Geometry: final body of the model. Coordinates: model frame, mm. A direction names the side the tool comes from. Coordinates: 2 decimals unless noted, no trailing zeros. Loops run counter-clockwise (first coordinate to the right, second up) from the corner with the lowest first, then second, coordinate; pieces in that order, holes last. Notation, with made-up numbers: (74.5, -36) - (81.5, -36) arc R16 ccw to (81.5, -21) - close; hole circle Ø7 at (45, 75). An arc over 180 degrees is marked (long way). Write each question's results on one line, items separated by ' | '. Start each with the question number.
from build123d import *

# Parameters (mm, degrees)
SKETCH1_W               = 12
SKETCH1_H               = 12
SKETCH1_R               = 5.5
BOSS_EXTRUDE1_DEPTH     = 6
BOSS_EXTRUDE1_2_DEPTH   = 6
BOSS_EXTRUDE1_3_DEPTH   = 6
BOSS_EXTRUDE1_4_DEPTH   = 6
BOSS_EXTRUDE1_5_DEPTH   = 6
BOSS_EXTRUDE1_6_DEPTH   = 6
BOSS_EXTRUDE2_START     = -6
BOSS_EXTRUDE2_OUTLINE_R = 1.7
BOSS_EXTRUDE2_DEPTH     = 6
CUT_EXTRUDE1_DEPTH      = 1


# Read off the part's stored shape, not the designer's step: Boss-Extrude2
with BuildPart() as part:
    # Sketch1 → Boss-Extrude1 (new body)
    with BuildSketch(Plane(origin=(0, 0, 0), x_dir=(1, 0, 0), z_dir=(0, 1, 0))):
        with Locations((-2.713611414, -10.664883528)):
            Rectangle(SKETCH1_W, SKETCH1_H)
        with Locations(Location((-2.713611414, -10.664883528, 0), (0, 0, 270))):
            Circle(SKETCH1_R, mode=Mode.SUBTRACT)
    extrude(amount=-BOSS_EXTRUDE1_DEPTH)



with BuildPart() as body_2:
    # Sketch1 → Boss-Extrude1 2 (new body)
    with BuildSketch(Plane(origin=(0, 0, 0), x_dir=(1, 0, 0), z_dir=(0, 1, 0))):
        with Locations((12.886388586, -10.664882884)):
            Rectangle(SKETCH1_W, SKETCH1_H)
        with Locations(Location((12.886388586, -10.664882884, 0), (0, 0, 270))):
            Circle(SKETCH1_R, mode=Mode.SUBTRACT)
    extrude(amount=-BOSS_EXTRUDE1_2_DEPTH)


with BuildPart() as body_3:
    # Sketch1 → Boss-Extrude1 3 (new body)
    with BuildSketch(Plane(origin=(0, 0, 0), x_dir=(1, 0, 0), z_dir=(0, 1, 0))):
        with Locations((5.086388588, -23.66488245)):
            Rectangle(SKETCH1_W, SKETCH1_H)
        with Locations(Location((5.086388588, -23.66488245, 0), (0, 0, 270))):
            Circle(SKETCH1_R, mode=Mode.SUBTRACT)
    extrude(amount=-BOSS_EXTRUDE1_3_DEPTH)


with BuildPart() as body_4:
    # Sketch1 → Boss-Extrude1 4 (new body)
    with BuildSketch(Plane(origin=(0, 0, 0), x_dir=(1, 0, 0), z_dir=(0, 1, 0))):
        with Locations((20.686388588, -23.664882884)):
            Rectangle(SKETCH1_W, SKETCH1_H)
        with Locations(Location((20.686388588, -23.664882884, 0), (0, 0, 270))):
            Circle(SKETCH1_R, mode=Mode.SUBTRACT)
    extrude(amount=-BOSS_EXTRUDE1_4_DEPTH)


with BuildPart() as body_5:
    # Sketch1 → Boss-Extrude1 5 (new body)
    with BuildSketch(Plane(origin=(0, 0, 0), x_dir=(1, 0, 0), z_dir=(0, 1, 0))):
        with Locations((28.486388586, -10.664882884)):
            Rectangle(SKETCH1_W, SKETCH1_H)
        with Locations(Location((28.486388586, -10.664882884, 0), (0, 0, 270))):
            Circle(SKETCH1_R, mode=Mode.SUBTRACT)
    extrude(amount=-BOSS_EXTRUDE1_5_DEPTH)


with BuildPart() as body_6:
    # Sketch1 → Boss-Extrude1 6 (new body)
    with BuildSketch(Plane(origin=(0, 0, 0), x_dir=(1, 0, 0), z_dir=(0, 1, 0))):
        with Locations((36.286388588, -23.664883087)):
            Rectangle(SKETCH1_W, SKETCH1_H)
        with Locations(Location((36.286388588, -23.664883087, 0), (0, 0, 270))):
            Circle(SKETCH1_R, mode=Mode.SUBTRACT)
    extrude(amount=-BOSS_EXTRUDE1_6_DEPTH)


with BuildPart() as part_1:
    add(part.part)

    add(body_2.part)  # Boss-Extrude2 merges body 2

    add(body_3.part)  # Boss-Extrude2 merges body 3

    add(body_4.part)  # Boss-Extrude2 merges body 4

    add(body_5.part)  # Boss-Extrude2 merges body 5

    add(body_6.part)  # Boss-Extrude2 merges body 6
    # Boss-Extrude2 outline → Boss-Extrude2 (add)
    with BuildSketch(Plane(origin=(0, 0, 0), x_dir=(1, 0, 0), z_dir=(0, 1, 0)).offset(BOSS_EXTRUDE2_START)):
        Polygon((23.186388588, -30.164882884), (33.786388588, -30.164882884), (33.786388588, -29.664883087), (30.286388588, -29.664883087), (30.286388588, -17.664883087), (42.286388588, -17.664883087), (42.286388588, -29.664883087), (38.786388588, -29.664883087), (38.786388588, -30.164883087), (54.418988347, -30.16488245), (54.418988347, -4.164883528), (30.986388586, -4.164882884), (30.986388586, -4.664882884), (34.486388586, -4.664882884), (34.486388586, -16.664882884), (22.486388586, -16.664882884), (22.486388586, -4.664882884), (25.986388586, -4.664882884), (25.986388586, -4.164882884), (15.386388586, -4.164882884), (15.386388586, -4.664882884), (18.886388586, -4.664882884), (18.886388586, -16.664882884), (6.886388586, -16.664882884), (6.886388586, -4.664882884), (10.386388586, -4.664882884), (10.386388586, -4.164882884), (-0.213611414, -4.164883528), (-0.213611414, -4.664883528), (3.286388586, -4.664883528), (3.286388586, -16.664883528), (-8.713611414, -16.664883528), (-8.713611414, -4.664883528), (-5.213611414, -4.664883528), (-5.213611414, -4.164883528), (-19.213611414, -4.164883528), (-19.213611414, -30.16488245), (2.586388588, -30.16488245), (2.586388588, -29.66488245), (-0.913611412, -29.66488245), (-0.913611412, -17.66488245), (11.086388588, -17.66488245), (11.086388588, -29.66488245), (7.586388588, -29.66488245), (7.586388588, -30.16488245), (18.186388588, -30.164882884), (18.186388588, -29.664882884), (14.686388588, -29.664882884), (14.686388588, -17.664882884), (26.686388588, -17.664882884), (26.686388588, -29.664882884), (23.186388588, -29.664882884), align=None)
        with Locations((-14.213611414, -17.164882989)):
            Circle(BOSS_EXTRUDE2_OUTLINE_R, mode=Mode.SUBTRACT)
        with Locations((49.418988347, -17.164882989)):
            Circle(BOSS_EXTRUDE2_OUTLINE_R, mode=Mode.SUBTRACT)
    extrude(amount=BOSS_EXTRUDE2_DEPTH)

    # Sketch2 → Cut-Extrude1 (cut)
    with BuildSketch(Plane(origin=(0, -6, 0), x_dir=(-1, 0, 0), z_dir=(0, -1, 0))):
        Polygon((6.798219501, -22.292392997), (8.345014372, -22.292392997), (8.345014372, -22.618034023), (7.083155398, -22.618034023), (7.083155398, -23.5949571), (8.345014372, -23.5949571), (8.345014372, -23.920598125), (7.083155398, -23.920598125), (7.083155398, -25.467392997), (6.798219501, -25.467392997), align=None)
        with BuildLine():
            Line((10.624501552, -22.292392997), (10.624501552, -22.618034023))
            Line((10.624501552, -22.618034023), (9.545179637, -22.618034023))
            Line((9.545179637, -22.618034023), (9.373454877, -23.453125169))
            add(Edge.make_bspline(
                [(9.373454877, -23.453125169), (9.407069849, -23.443844851), (9.47219354, -23.425865702), (9.568314271, -23.405903325), (9.65956577, -23.393869672), (9.718779856, -23.392226555), (9.747433243, -23.391431459)],
                knots=[0, 0, 0, 0, 1.100273476, 2.13160584, 3.095893838, 4, 4, 4, 4], degree=3))
            add(Edge.make_bspline(
                [(9.747433243, -23.391431459), (9.782887778, -23.392198843), (9.852600253, -23.393707713), (9.95459844, -23.408196462), (10.051964708, -23.431001956), (10.144495429, -23.462861287), (10.232361786, -23.50360083), (10.314755359, -23.55449149), (10.392912895, -23.613939584), (10.465432248, -23.682288273), (10.531222156, -23.757510025), (10.589067018, -23.838388951), (10.638200225, -23.924139045), (10.677716053, -24.015579597), (10.709270413, -24.111699686), (10.73027258, -24.213510672), (10.744257737, -24.320052895), (10.745820188, -24.392900612), (10.746616936, -24.430048246)],
                knots=[0, 0, 0, 0, 1.052922333, 2.070308379, 3.05430497, 4.020497103, 4.973039431, 5.925935799, 6.892292201, 7.88610001, 8.88166317, 9.857072816, 10.836096531, 11.812156883, 12.81219415, 13.836441305, 14.89672472, 16, 16, 16, 16], degree=3))
            add(Edge.make_bspline(
                [(10.746616936, -24.430048246), (10.746013618, -24.455921974), (10.744815135, -24.50731977), (10.738720416, -24.583650581), (10.726985874, -24.658365436), (10.711230867, -24.731474249), (10.690781673, -24.802838608), (10.666026603, -24.87266278), (10.635731635, -24.940512173), (10.602501745, -25.007028781), (10.565085297, -25.070708856), (10.523557651, -25.130261865), (10.479683241, -25.186581177), (10.43247427, -25.239062778), (10.381491939, -25.287361801), (10.327353683, -25.331764885), (10.270491502, -25.373022949), (10.210025675, -25.409461241), (10.147303566, -25.442991922), (10.081419397, -25.470499703), (10.013872905, -25.495092824), (9.94369191, -25.514695753), (9.87103538, -25.530055999), (9.795783548, -25.540488687), (9.718331083, -25.548087312), (9.665830179, -25.548562979), (9.639310246, -25.548803254)],
                knots=[0, 0, 0, 0, 1.056347294, 2.098418968, 3.122841568, 4.141288669, 5.149314143, 6.15115421, 7.162517403, 8.180376062, 9.185164535, 10.17417709, 11.141909838, 12.097768115, 13.052685741, 14.0056014, 14.954263652, 15.917497458, 16.885230207, 17.854509472, 18.828990115, 19.81800267, 20.826176721, 21.857883937, 22.917946725, 24, 24, 24, 24], degree=3))
            add(Edge.make_bspline(
                [(9.639310246, -25.548803254), (9.607674382, -25.548176565), (9.545434557, -25.546943629), (9.454248042, -25.534045431), (9.366514079, -25.51557245), (9.282938915, -25.487780977), (9.202773555, -25.452958217), (9.127097232, -25.408947118), (9.053976278, -25.359073217), (8.986383216, -25.300217468), (8.923648742, -25.235886814), (8.867490695, -25.166075239), (8.817476664, -25.09193496), (8.774407565, -25.01310592), (8.737670075, -24.929795253), (8.708809335, -24.841690816), (8.685515399, -24.749252955), (8.675660725, -24.685613699), (8.670655398, -24.653290433)],
                knots=[0, 0, 0, 0, 1.0467383, 2.05933395, 3.04377827, 4.011590433, 4.970194871, 5.932262533, 6.905835911, 7.896367577, 8.894135286, 9.877477877, 10.858688626, 11.851381753, 12.8477658, 13.868841284, 14.917554742, 16, 16, 16, 16], degree=3))
            Line((8.670655398, -24.653290433), (8.955591295, -24.653290433))
            add(Edge.make_bspline(
                [(8.955591295, -24.653290433), (8.962602201, -24.683567644), (8.976077551, -24.741762123), (9.005655623, -24.823524126), (9.041819667, -24.896385136), (9.084822183, -24.961308972), (9.13612114, -25.017922848), (9.19465855, -25.068375469), (9.26028827, -25.113891479), (9.333216414, -25.151830703), (9.410153993, -25.184187358), (9.490678534, -25.205733539), (9.572597477, -25.220883634), (9.628004284, -25.22240016), (9.655846704, -25.223162228)],
                knots=[0, 0, 0, 0, 1.136247022, 2.183929868, 3.172523383, 4.106158343, 5.02341133, 5.958108904, 6.928429099, 7.938127109, 8.96079061, 9.975095812, 10.982467395, 12, 12, 12, 12], degree=3))
            add(Edge.make_bspline(
                [(9.655846704, -25.223162228), (9.683023293, -25.222417665), (9.736534219, -25.220951615), (9.815284548, -25.209667654), (9.891314798, -25.192289), (9.963874758, -25.166281346), (10.034234154, -25.134672208), (10.100613217, -25.094109247), (10.164932256, -25.047427659), (10.225192063, -24.993945573), (10.280382135, -24.935008778), (10.329146616, -24.871982857), (10.369765673, -24.804748289), (10.4039959, -24.734469072), (10.429988536, -24.660374952), (10.448531426, -24.582813172), (10.459419915, -24.501592154), (10.460917771, -24.446193566), (10.461681039, -24.417963911)],
                knots=[0, 0, 0, 0, 1.027316725, 2.022795036, 3.002884548, 3.971462791, 4.93288096, 5.914575861, 6.907176829, 7.935150275, 8.956128384, 9.956726525, 10.942570165, 11.921478529, 12.907843606, 13.90538589, 14.932640048, 16, 16, 16, 16], degree=3))
            add(Edge.make_bspline(
                [(10.461681039, -24.417963911), (10.461083704, -24.392495193), (10.459914506, -24.342643802), (10.450361774, -24.269710237), (10.433745664, -24.20070112), (10.410682573, -24.135283207), (10.381400448, -24.073394799), (10.345617007, -24.014972023), (10.302660711, -23.960784903), (10.25359164, -23.910808086), (10.199836132, -23.864684521), (10.140469308, -23.825365243), (10.076733517, -23.79228726), (10.009396666, -23.76374129), (9.93685708, -23.743239186), (9.860551277, -23.72784689), (9.779655264, -23.718942953), (9.72434614, -23.717707526), (9.695915815, -23.717072484)],
                knots=[0, 0, 0, 0, 1.045622112, 2.046656509, 3.013763289, 3.955457236, 4.890082067, 5.820317437, 6.762574623, 7.722996705, 8.69280354, 9.665887285, 10.63943826, 11.638615906, 12.663482002, 13.728887084, 14.832589034, 16, 16, 16, 16], degree=3))
            add(Edge.make_bspline(
                [(9.695915815, -23.717072484), (9.671306001, -23.717599164), (9.620492978, -23.718686622), (9.5425487, -23.726693516), (9.460641208, -23.73961059), (9.375084487, -23.757378115), (9.285621598, -23.780629163), (9.192441334, -23.808491603), (9.095347778, -23.841803701), (9.0299267, -23.866960781), (8.996296424, -23.879892997)],
                knots=[0, 0, 0, 0, 0.817624296, 1.688186739, 2.600797293, 3.572016777, 4.590301741, 5.671205678, 6.80286297, 8, 8, 8, 8], degree=3))
            Line((8.996296424, -23.879892997), (9.321937449, -22.292392997))
            Line((9.321937449, -22.292392997), (10.624501552, -22.292392997))
        make_face()
    extrude(amount=-CUT_EXTRUDE1_DEPTH, mode=Mode.SUBTRACT)


solid = part_1.part
1) Material intervals for line 1 (X direction, y = -3.75, z = 23.75); line 2 (X direction, y = -0.5, z = 15); line 3 (Z direction, x = 2, y = -4.5), sorted ascending. Write a range as [from, to].
2) Section query A-A on z = 27.5. Output: boundary loops of the cut face in (x, y).
3) Section query C-C on z = 11.5. Output: boundary loops of the cut face in (x, y), and give its area (3 significant figures).
4) Section query D-D on y = -1.5. Count the separate pieces of the cut face and the enclosed holes in it, and give its area (3 significant figures).
5) Pull-direction query (Z, two-part tool) for faces 1 (the flat face through (17, -6, 17)), 2 (the flat face through (-9.87, -5, 23.55)), 3 (the flat face through (21, -3, 29.665)), 4 (the flat face through (43, -3, 4.165)); classes: released by +Z, released by -Z, zero draft, split by the parting line, or undercut.
6) Section query B-B on x = 6. Output: boundary loops of the cut face in (y, z).
7) Access query for faces 5 (the flat face through (-12, -3, 4.165)), 6 (the flat face through (36, -3, 29.665)). Directions: +Z, -Z, +X, -X, +Y, -Y. A direction counts if a zero-diameter tool reaches every point of the face in a straight line with its end or side. Return the directions, or none.
8) Pin query (flat end, axial travel): pin 1 Ø4.5 at (x, z) = (-14.21, 17.16) entering from -Y; pin 2 Ø1.5 at (x, y) = (-1.5, -3) entering from -Z. Return the tip coordinate at first contact, or that it passes through.
Returned:
1) line 1: x = [-19.21, -0.41], [10.59, 15.19], [26.19, 30.79], [41.79, 54.42] | line 2: x = [-19.21, -6.1], [0.67, 9.5], [16.27, 25.1], [31.87, 54.42] | line 3: z = [4.16, 7.83], [13.5, 19.11], [28.22, 30.16]
2) outline: (-19.21, -6) - (1.14, -6) - (1.14, 0) - (-19.21, 0) - close; (9.03, -6) - (16.74, -6) - (16.74, 0) - (9.03, 0) - close; (24.63, -6) - (32.34, -6) - (32.34, 0) - (24.63, 0) - close; (40.23, -6) - (54.42, -6) - (54.42, 0) - (40.23, 0) - close
3) outline: (-19.21, -6) - (-8.15, -6) - (-8.15, 0) - (-19.21, 0) - close; (2.72, -6) - (7.45, -6) - (7.45, 0) - (2.72, 0) - close; (18.32, -6) - (23.05, -6) - (23.05, 0) - (18.32, 0) - close; (33.92, -6) - (54.42, -6) - (54.42, 0) - (33.92, 0) - close | area: 246 mm²
4) separate pieces: 1 | enclosed holes: 8 | area: 1,310 mm²
5) face 1: zero draft | face 2: undercut | face 3: released by +Z | face 4: released by -Z
6) outline: (-6, 4.16) - (0, 4.16) - (0, 18.24) - (-6, 18.24) - close; (-6, 29.09) - (0, 29.09) - (0, 29.66) - (-6, 29.66) - close
7) face 5: -Z, +X, -X, +Y, -Y | face 6: +Z, +Y, -Y
8) pin 1: stops at y = -6 | pin 2: stops at z = 4.66
